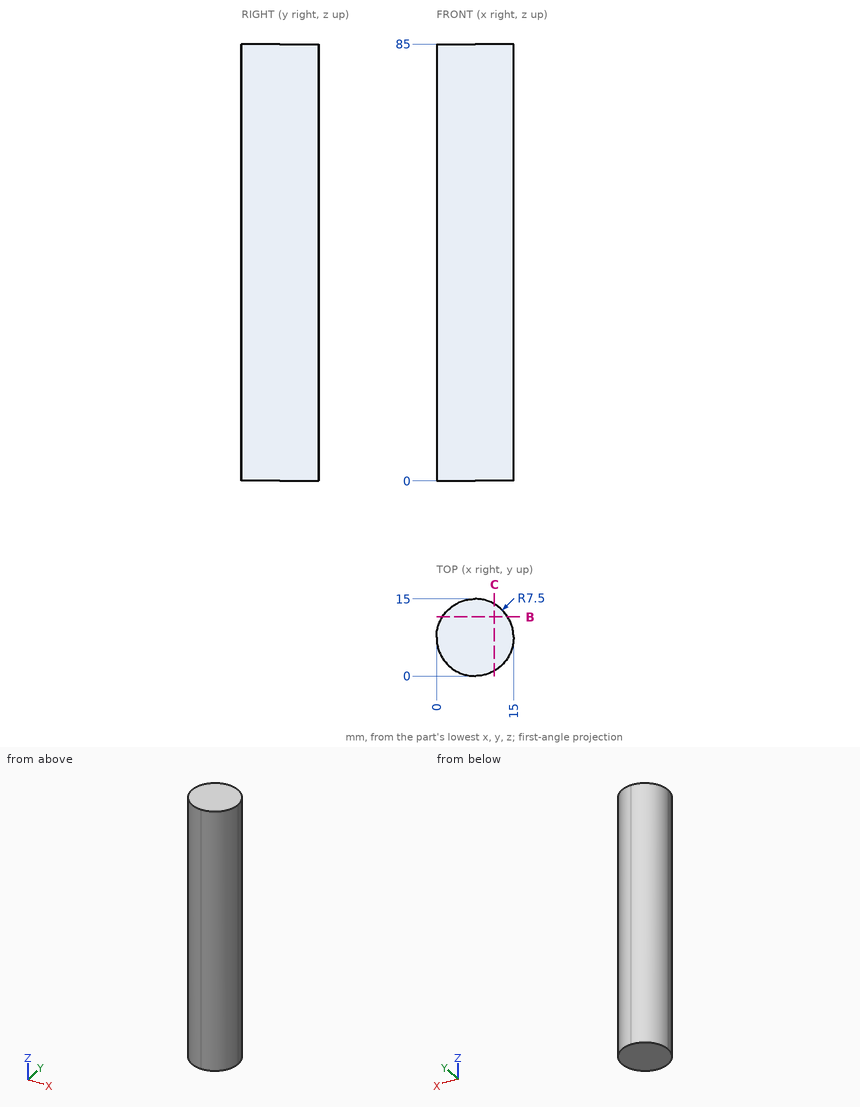
Job drawing, mm, ordinate dimensions from the low corner. One solid piece. Give positions to 0.01 mm unless a question says otherwise; leave off trailing zeros. Order: outer loops, then holes, each group sorted by start corner. A loop starts at its lowest first (then second) coordinate and runs counter-clockwise, first axis right, second up. Notation, with made-up numbers: (-10, 33.5) - (15, 33.5) arc R29 cw to (15, 61.5) - close; hole circle Ø7 at (62.5, 89). An arc over 180 degrees is marked (long way). Answer in a Markdown table with one row per item.
1. Probe probe 1 along Y at (x, z) = (7.25, 5.5); probe 2 along Y at (x, z) = (12.5, 58.5); probe 3 along X at (y, z) = (3.75, 48). List the from-to ranges inside material, lowest first. Write a range as [from, to].
Data:
| item | result |
|---|---|
| probe 1 | y = [0, 15] |
| probe 2 | y = [1.91, 13.09] |
| probe 3 | x = [1, 14] |
2. Saw through at C-C, the plane x = 11.25. Give the cut face in (y, z), plus the area to 3 significant figures.
Data:
| item | result |
|---|---|
| outline | (1, 0) - (14, 0) - (14, 85) - (1, 85) - close |
| area | 1,100 mm² |
3. Saw through at B-B, the plane y = 11.5. Give the cut face in (x, z), plus the area to 3 significant figures.
Data:
| item | result |
|---|---|
| outline | (1.16, 0) - (13.84, 0) - (13.84, 85) - (1.16, 85) - close |
| area | 1,080 mm² |
4. Flat gauge pins, fed straight in: pin 1 (8 mm diameter, centred on x = 4, z = 27, fed in from +Y); pin 2 (6 mm diameter, centred on y = 2.5, z = 43.5, fed in from +X); pin 3 (1.5 mm diameter, centred on x = 11, z = 31.5, fed in from +Y); pin 4 (6 mm diameter, centred on y = 1.5, z = 20.5, fed in from +X). Where does each tip first touch, or does it go through?
Data:
| item | result |
|---|---|
| pin 1 | stops at y = 15 |
| pin 2 | stops at x = 14.73 |
| pin 3 | stops at y = 14.48 |
| pin 4 | stops at x = 14.37 |
